The model under review builds one solid part; all positions refer to its coordinate system, in mm. Face numbers are marked on the shaded views. Round coordinates to 2 decimals unless told otherwise and drop trailing zeros. Order: outer loops, then holes, each group sorted by start corner. A loop starts at its lowest first (then second) coordinate and runs counter-clockwise, first axis right, second up. Notation, with made-up numbers: M 77,86.25 L 81,86.25 A21 cw 81,118.25 Z; hole C 68,69.25 d8. An arc over 180 degrees is marked long. Answer as a JSON object with one key per item and string values. Group by question number.
1) Consider section D-D, the plane y = -17. Write out the cut boundary in (x, z).
2) The part is to be moulded in two halves that separate along X. For the marked faces 1, 2 and 3, say which applies: +X half, -X half, draft (parallel to the pull), parting line (faces both ways), or undercut.
3) Consider section C-C, the plane x = -7.5. Write out the cut boundary in (y, z).
4) Consider section B-B, the plane z = 70. Write out the cut boundary in (x, y).
5) Consider section A-A, the plane y = -28. Write out the cut boundary in (x, z), then the cut area to 3 significant figures.
6) Insertion check: pin 1 Ø6 at (x, z) = (-4, 98.5) entering from -Y; pin 2 Ø1 at (y, z) = (-11.5, 92) entering from -X; pin 3 Ø6 at (x, z) = (-44, 29) entering from +Y; pin 4 Ø4 at (x, y) = (-3.5, -34) entering from +Z. Each pin has a flat end and moves straight along its axis. Give the tip position at first contact, or say it passes through.
7) To check wall thickness, follow line 1 (Z direction, x = -23, y = -18); line 2 (Z direction, x = -39, y = -9.5); line 3 (Y direction, x = -28.5, z = 50). State the ranges of each line that lie inside material, in increasing order.
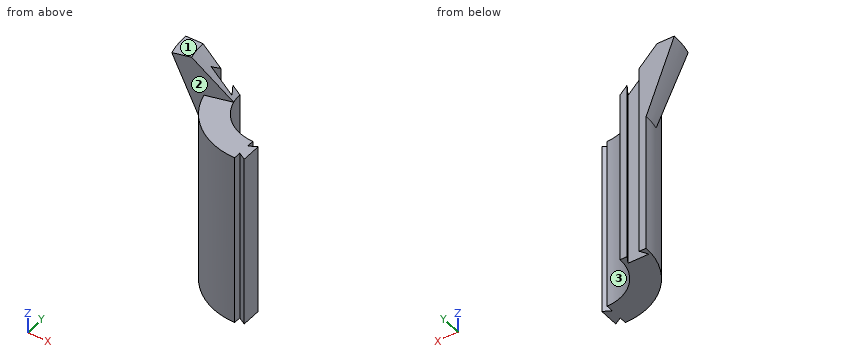
```python
from build123d import *

# Parameters (mm, degrees)
BOSS_EXTRUDE2_DEPTH     = 100
REVOLVE1_ANGLE          = 14.32
CUT_EXTRUDE2_DEPTH      = 140.472452218
CUT_EXTRUDE2_DEPTH_BACK = 140.472452218
BOSS_EXTRUDE4_DEPTH     = 100


with BuildPart() as part:
    # Sketch1 → Boss-Extrude2 (new body)
    with BuildSketch(Plane.XY):
        with BuildLine():
            Line((-40, 0), (-25, 0))
            ThreePointArc((-25, 0), (-17.67766953, -17.67766953), (0, -25))
            Line((0, -25), (0, -40))
            ThreePointArc((0, -40), (-28.284271247, -28.284271247), (-40, 0))
        make_face()
    extrude(amount=BOSS_EXTRUDE2_DEPTH)

    # Sketch2 → Revolve1 (revolve)
    with BuildSketch(Plane(origin=(0, 0, 0), x_dir=(1, 0, 0), z_dir=(0, 1, 0))):
        Polygon((-25, -100), (-46.213203436, -121.213203436), (-56.213203436, -121.213203436), (-40, -80), align=None)
    revolve(axis=Axis((0, 0, 0), (0, 0, 1)), revolution_arc=REVOLVE1_ANGLE)

    # Sketch4 → Cut-Extrude2 (cut, two sides: drawn at the far end of the back side and taken through both)
    with BuildSketch(Plane(origin=(0, 0, 0), x_dir=(-1, 0, 0), z_dir=(0, 0, -1)).offset(-CUT_EXTRUDE2_DEPTH_BACK)):
        Polygon((-98.13708499, 0), (25, 0), (29, 0), (26.5, -4.330127019), (38.5, -4.330127019), (36, 0), (40, 0), (163.13708499, 0), (163.13708499, 246.27416998), (-98.13708499, 246.27416998), align=None)
    extrude(amount=CUT_EXTRUDE2_DEPTH + CUT_EXTRUDE2_DEPTH_BACK, mode=Mode.SUBTRACT)

    # Sketch5 → Boss-Extrude4 (add)
    with BuildSketch(Plane(origin=(0, 0, 0), x_dir=(-1, 0, 0), z_dir=(0, 0, -1))):
        Polygon((0, -35.75), (0, -29.25), (-4.330127019, -26.75), (-4.330127019, -38.25), align=None)
    extrude(amount=-BOSS_EXTRUDE4_DEPTH)


solid = part.part
```
Results list:
{
 "1": {"outline": "M -36.21,0 L -18.33,0 L -18.33,100 L -36.21,100 Z"},
 "2": {"face 1": "draft", "face 2": "undercut", "face 3": "+X half"},
 "3": {"outline": "M -39.29,0 L -23.85,0 L -23.85,100 L -39.29,100 Z"},
 "4": {"outline": "M -40,0 A40 ccw 0,-40 L 0,-35.75 L 4.33,-38.25 L 4.33,-26.75 L 0,-29.25 L 0,-25 A25 cw -25,0 L -29,0 L -26.5,-4.33 L -38.5,-4.33 L -36,0 Z"},
 "5": {"outline": "M -28.57,0 L 0,0 L 0,100 L -28.57,100 Z; M 2.17,0 L 4.33,0 L 4.33,100 L 2.17,100 Z", "area": "3,070 mm^2"},
 "6": {"pin 1": "y = -39.99", "pin 2": "x = -43.44", "pin 3": "through", "pin 4": "z = 100"},
 "7": {"line 1": "0 to 100", "line 2": "80.36 to 115.14", "line 3": "-28.07 to -4.33, -0.87 to 0"}
}
